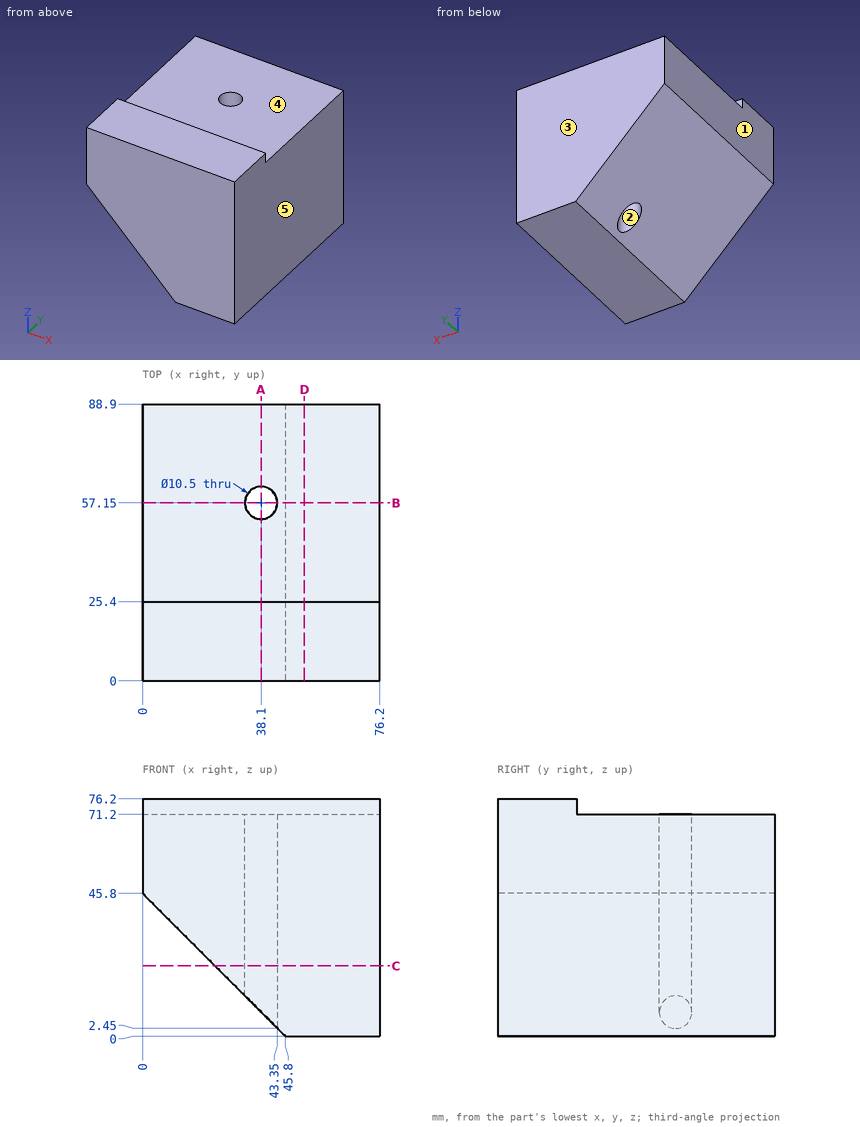
Geometry check sheet. Reference: drawing and pictorial views, mm from the part's lowest x, y, z. A direction names the side the tool comes from. Coordinates: 2 decimals unless noted, no trailing zeros. Loops run counter-clockwise (first coordinate to the right, second up) from the corner with the lowest first, then second, coordinate; pieces in that order, holes last. Notation, with made-up numbers: (80.5, 31) -> (98.5, 31) arc R23 cw to (98.5, 60) -> close; hole circle Ø9 at (13, 78). An arc over 180 degrees is marked (long way). Write item = value, one per line. Start each with the question number.
1. Section check D-D on x = 52. Record the cut outline in (y, z), then the cut area to 3 significant figures.
2. Draft check along Y on the marked faces 1, 2 and 3. Enter one of: released by +Y, released by -Y, zero draft, split by the parting line, or undercut.
3. Material ranges on line 1 (Y direction, x = 38.1, z = 53); line 2 (Z direction, x = 63.5, y = 80); line 3 (X direction, y = 57.15, z = 39), recorded low to high.
4. Section check A-A on x = 38.1. Record the cut outline in (y, z), then the cut area to 3 significant figures.
5. Tool access check on the marked faces 4 and 5. Record the directions out of +Z, -Z, +X, -X, +Y, -Y that give a thin tool (end or side, any length) a straight path to the whole face; none if there is none.
6. Section check B-B on y = 57.15. Record the cut outline in (x, z), then the cut area to 3 significant figures.
7. Depth check by flat-ended pin: P1, Ø5, axis at x = 26, y = 78.5, coming from the -Z side; P2, Ø4, axis at x = 21, y = 28.5, coming from the -Z side; P3, Ø12, axis at x = 38.1, y = 57.15, coming from the +Z side. Enter the tip coordinate at first touch or a pass-through.
8. Section check C-C on z = 22.5. Record the cut outline in (x, y).
Responses:
q1.outline = (0, 0) -> (88.9, 0) -> (88.9, 71.2) -> (25.4, 71.2) -> (25.4, 76.2) -> (0, 76.2) -> close
q1.area = 6,460 mm2
q2.face_1 = zero draft
q2.face_2 = undercut
q2.face_3 = released by +Y
q3.line_1 = 0 to 51.9, 62.4 to 88.9
q3.line_2 = 0 to 71.2
q3.line_3 = 6.8 to 32.85, 43.35 to 76.2
q4.outline = (0, 7.7) -> (51.9, 7.7) -> (51.9, 71.2) -> (25.4, 71.2) -> (25.4, 76.2) -> (0, 76.2) -> close; (62.4, 7.7) -> (88.9, 7.7) -> (88.9, 71.2) -> (62.4, 71.2) -> close
q4.area = 5,110 mm2
q5.face_4 = +Z, +X, -X, +Y
q5.face_5 = +Z, -Z, +X, +Y, -Y
q6.outline = (0, 45.8) -> (32.85, 12.95) -> (32.85, 71.2) -> (0, 71.2) -> close; (43.35, 2.45) -> (45.8, 0) -> (76.2, 0) -> (76.2, 71.2) -> (43.35, 71.2) -> close
q6.area = 3,710 mm2
q7.P1 = 17.3
q7.P2 = 22.8
q7.P3 = 71.2
q8.outline = (23.3, 0) -> (76.2, 0) -> (76.2, 88.9) -> (23.3, 88.9) -> close; hole circle Ø10.5 at (38.1, 57.15)
